from build123d import *

# Parameters (mm, degrees)
SKETCH1_W           = 75
SKETCH1_H           = 75
SKETCH1_R           = 1.25
BOSS_EXTRUDE1_DEPTH = 5
SKETCH2_W           = 75
SKETCH2_H           = 5
BOSS_EXTRUDE2_DEPTH = 10
CUT_EXTRUDE1_REACH  = 87.184
SKETCH3_R           = 1.25


with BuildPart() as part:
    # Sketch1 → Boss-Extrude1 (new body)
    with BuildSketch(Plane.XY):
        Rectangle(SKETCH1_W, SKETCH1_H)
        with Locations((-25.25, -30)):
            Circle(SKETCH1_R, mode=Mode.SUBTRACT)
        with Locations((-15.25, -30)):
            Circle(SKETCH1_R, mode=Mode.SUBTRACT)
        with Locations((-5.25, -30)):
            Circle(SKETCH1_R, mode=Mode.SUBTRACT)
        with Locations((4.75, -30)):
            Circle(SKETCH1_R, mode=Mode.SUBTRACT)
        with Locations((14.75, -30)):
            Circle(SKETCH1_R, mode=Mode.SUBTRACT)
        with Locations((24.75, -30)):
            Circle(SKETCH1_R, mode=Mode.SUBTRACT)
    extrude(amount=BOSS_EXTRUDE1_DEPTH)

    # Sketch2 → Boss-Extrude2 (add)
    with BuildSketch(Plane.XY.offset(5)):
        with Locations((0, 35)):
            Rectangle(SKETCH2_W, SKETCH2_H)
    extrude(amount=BOSS_EXTRUDE2_DEPTH)

    # Sketch3 → Cut-Extrude1 (cut, up to next)
    with BuildSketch(Plane(origin=(0, 37.5, 0), x_dir=(1, 0, 0), z_dir=(0, 1, 0)), mode=Mode.PRIVATE) as cut_extrude1_sk1:
        with Locations(Location((-25.25, -9, 0), (0, 0, 270))):
            Circle(SKETCH3_R)
    cut_extrude1_tool1 = extrude(cut_extrude1_sk1.sketch, amount=-CUT_EXTRUDE1_REACH, mode=Mode.PRIVATE) & part.part
    # Sketch3 → Cut-Extrude1 (cut, up to next)
    with BuildSketch(Plane(origin=(0, 37.5, 0), x_dir=(1, 0, 0), z_dir=(0, 1, 0)), mode=Mode.PRIVATE) as cut_extrude1_sk2:
        with Locations(Location((-15.25, -9, 0), (0, 0, 270))):
            Circle(SKETCH3_R)
    cut_extrude1_tool2 = extrude(cut_extrude1_sk2.sketch, amount=-CUT_EXTRUDE1_REACH, mode=Mode.PRIVATE) & part.part
    # Sketch3 → Cut-Extrude1 (cut, up to next)
    with BuildSketch(Plane(origin=(0, 37.5, 0), x_dir=(1, 0, 0), z_dir=(0, 1, 0)), mode=Mode.PRIVATE) as cut_extrude1_sk3:
        with Locations(Location((-5.25, -9, 0), (0, 0, 270))):
            Circle(SKETCH3_R)
    cut_extrude1_tool3 = extrude(cut_extrude1_sk3.sketch, amount=-CUT_EXTRUDE1_REACH, mode=Mode.PRIVATE) & part.part
    # Sketch3 → Cut-Extrude1 (cut, up to next)
    with BuildSketch(Plane(origin=(0, 37.5, 0), x_dir=(1, 0, 0), z_dir=(0, 1, 0)), mode=Mode.PRIVATE) as cut_extrude1_sk4:
        with Locations(Location((4.75, -9, 0), (0, 0, 270))):
            Circle(SKETCH3_R)
    cut_extrude1_tool4 = extrude(cut_extrude1_sk4.sketch, amount=-CUT_EXTRUDE1_REACH, mode=Mode.PRIVATE) & part.part
    # Sketch3 → Cut-Extrude1 (cut, up to next)
    with BuildSketch(Plane(origin=(0, 37.5, 0), x_dir=(1, 0, 0), z_dir=(0, 1, 0)), mode=Mode.PRIVATE) as cut_extrude1_sk5:
        with Locations(Location((14.75, -9, 0), (0, 0, 270))):
            Circle(SKETCH3_R)
    cut_extrude1_tool5 = extrude(cut_extrude1_sk5.sketch, amount=-CUT_EXTRUDE1_REACH, mode=Mode.PRIVATE) & part.part
    # Sketch3 → Cut-Extrude1 (cut, up to next)
    with BuildSketch(Plane(origin=(0, 37.5, 0), x_dir=(1, 0, 0), z_dir=(0, 1, 0)), mode=Mode.PRIVATE) as cut_extrude1_sk6:
        with Locations(Location((24.75, -9, 0), (0, 0, 270))):
            Circle(SKETCH3_R)
    cut_extrude1_tool6 = extrude(cut_extrude1_sk6.sketch, amount=-CUT_EXTRUDE1_REACH, mode=Mode.PRIVATE) & part.part
    add(cut_extrude1_tool1.solids().sort_by_distance((-25.25, 37.5, 9))[0], mode=Mode.SUBTRACT)
    add(cut_extrude1_tool2.solids().sort_by_distance((-15.25, 37.5, 9))[0], mode=Mode.SUBTRACT)
    add(cut_extrude1_tool3.solids().sort_by_distance((-5.25, 37.5, 9))[0], mode=Mode.SUBTRACT)
    add(cut_extrude1_tool4.solids().sort_by_distance((4.75, 37.5, 9))[0], mode=Mode.SUBTRACT)
    add(cut_extrude1_tool5.solids().sort_by_distance((14.75, 37.5, 9))[0], mode=Mode.SUBTRACT)
    add(cut_extrude1_tool6.solids().sort_by_distance((24.75, 37.5, 9))[0], mode=Mode.SUBTRACT)


solid = part.part
Work out the finished part from the listing and answer in its coordinate system (mm). A direction names the side the tool comes from. Coordinates: 2 decimals unless noted, no trailing zeros. Loops run counter-clockwise (first coordinate to the right, second up) from the corner with the lowest first, then second, coordinate; pieces in that order, holes last. Notation, with made-up numbers: (63, -31.75) -> (79, -31.75) arc R13 ccw to (79, -26.75) -> close; hole circle Ø11 at (-5.75, 3.5). An arc over 180 degrees is marked (long way). Write each question's results on one line, items separated by ' | '. Start each with the question number.
1) For faces 1 (the cylindrical face through (15.595, 35.035, 8.079)), 2 (the flat face through (-1, 32.5, 10)), determine the directions among +Z, -Z, +X, -X, +Y, -Y from which every point of the face is accessible in a straight line to the end or side of a thin tool.
2) Find section A-A on z = 9. Determine the outline of the cut face in (x, y), then the cut area to 3 significant figures.
3) Find section C-C on y = -30. Determine the outline of the cut face in (x, z).
4) Find section D-D on y = -18. Determine the outline of the cut face in (x, z).
5) Find section B-B on x = 14.75. Determine the outline of the cut face in (y, z), then the cut area to 3 significant figures.
6) Flat-ended cylindrical pins translate along their axes: P1, Ø2, axis at x = -5.25, y = -30, coming from the -Z side; P2, Ø3, axis at x = -14, z = 12, coming from the -Y side; P3, Ø4, axis at x = 14.75, y = -30, coming from the +Z side. Find the tip coordinate at first contact, or state that the pin passes through.
7) Consider line 1 along Y through (x, z) = (-25.25, 1.8); line 2 along Z through (x, y) = (-15, 16.5); line 3 along Y through (x, z) = (-23, 10.25). Determine where each line is inside the solid, lowest interval first.
8) The mould has two halves that part along X. Classify faces 3 (the cylindrical face through (-16, -29, 2)), 4 (the flat face through (-1, 35, 15)), 5 (the flat face through (37.5, 8, 4)), 6 (the cylindrical face through (24.8, 35.03, 7.75)): pulls with the +X half, pulls with the -X half, needs draft (parallel to the pull), parting line crosses it, or undercut.
Response values:
1) face 1: +Y, -Y | face 2: +Z, +X, -X, -Y
2) outline: (-37.5, 32.5) -> (-26.5, 32.5) -> (-26.5, 37.5) -> (-37.5, 37.5) -> close; (-24, 32.5) -> (-16.5, 32.5) -> (-16.5, 37.5) -> (-24, 37.5) -> close; (-14, 32.5) -> (-6.5, 32.5) -> (-6.5, 37.5) -> (-14, 37.5) -> close; (-4, 32.5) -> (3.5, 32.5) -> (3.5, 37.5) -> (-4, 37.5) -> close; (6, 32.5) -> (13.5, 32.5) -> (13.5, 37.5) -> (6, 37.5) -> close; (16, 32.5) -> (23.5, 32.5) -> (23.5, 37.5) -> (16, 37.5) -> close; (26, 32.5) -> (37.5, 32.5) -> (37.5, 37.5) -> (26, 37.5) -> close | area: 300 mm^2
3) outline: (-37.5, 0) -> (-26.5, 0) -> (-26.5, 5) -> (-37.5, 5) -> close; (-24, 0) -> (-16.5, 0) -> (-16.5, 5) -> (-24, 5) -> close; (-14, 0) -> (-6.5, 0) -> (-6.5, 5) -> (-14, 5) -> close; (-4, 0) -> (3.5, 0) -> (3.5, 5) -> (-4, 5) -> close; (6, 0) -> (13.5, 0) -> (13.5, 5) -> (6, 5) -> close; (16, 0) -> (23.5, 0) -> (23.5, 5) -> (16, 5) -> close; (26, 0) -> (37.5, 0) -> (37.5, 5) -> (26, 5) -> close
4) outline: (-37.5, 0) -> (37.5, 0) -> (37.5, 5) -> (-37.5, 5) -> close
5) outline: (-37.5, 0) -> (-31.25, 0) -> (-31.25, 5) -> (-37.5, 5) -> close; (-28.75, 0) -> (37.5, 0) -> (37.5, 7.75) -> (32.5, 7.75) -> (32.5, 5) -> (-28.75, 5) -> close; (32.5, 10.25) -> (37.5, 10.25) -> (37.5, 15) -> (32.5, 15) -> close | area: 400 mm^2
6) P1: passes through | P2: stops at y = 32.5 | P3: stops at z = 5
7) line 1: y = -37.5 to -31.25, -28.75 to 37.5 | line 2: z = 0 to 5 | line 3: y = 32.5 to 37.5
8) face 3: undercut | face 4: needs draft | face 5: pulls with the +X half | face 6: undercut
